Autodesk Inventor part; units mm, degrees
ref_plane "body_to_body2_XY" through (0, -15.2908, 0) normal (0, -1, 0) x (1, 0, 0)
ref_plane "body_to_body2_YZ" through (0, -15.2908, 0) normal (1, 0, 0) x (0, 0, 1)
ref_plane "body_to_body2_ZX" through (0, -15.2908, 0) normal (0, 0, 1) x (0, -1, 0)
sketch "Sketch_1" plane through (0, 0, 0) normal (0, 1, 0) x (-1, 0, 0)
  line L0 (9.7028, 14.4018) -> (-9.7028, 14.4018)
  line L1 (-9.7028, 14.4018) -> (-9.7028, -14.4018)
  line L2 (-9.7028, -14.4018) -> (9.7028, -14.4018)
  line L3 (9.7028, -14.4018) -> (9.7028, 14.4018)
extrude "Extrusion1" add sketch "Sketch_1" against normal blind 22.3012
sketch "Sketch_2" plane through (0, 0, 0) normal (0, 1, 0) x (-1, 0, 0)
  circle A0 centre (0, 0) radius 8.5725
extrude "Extrusion2" add sketch "Sketch_2" along normal blind 0.9906
sketch "Sketch_3" plane through (0, 0, 0) normal (1, 0, 0) x (0, 1, 0)
  line L0 (0.9906, 0) -> (9.6012, 0)
  line L1 (9.6012, 0) -> (9.6012, -4.9265)
  line L2 (9.6012, -4.9265) -> (8.5277, -6)
  line L3 (8.5277, -6) -> (0.9906, -6)
  line L4 (0.9906, -6) -> (0.9906, 0)
  line L5 (0.9906, 0) -> (9.6012, 0)
revolve "Revolution1" add sketch "Sketch_3" angle 360 about axis through (0, 0.9906, 0) along (0, 1, 0)
sketch "Sketch_10" plane through (0, 0.9906, 0) normal (0, 1, 0) x (1, 0, 0)
  line L0 (-2.9909, 5.2014) -> (2.9909, 5.2014)
  arc A0 (2.9909, 5.2014) -> (-2.9909, 5.2014) centre (0, 0) ccw
extrude "Extrusion3" cut sketch "Sketch_10" along normal blind 8.6106
sketch "Sketch5" plane through (0, 9.6012, 0) normal (0, 1, 0) x (1, 0, 0)
  point P0 (0, 0)
hole "Drilling 1" at (0, 9.6012, 0) direction (0, -1, 0) diameter 6 depth 8.6106 countersink diameter 8 countersink angle 90
sketch "Sketch_5" plane through (0, -22.3012, 0) normal (0, 1, 0) x (1, 0, 0)
  line L0 (-8.4328, -13.1318) -> (8.4328, -13.1318)
  line L1 (8.4328, -13.1318) -> (8.4328, 13.1318)
  line L2 (8.4328, 13.1318) -> (-8.4328, 13.1318)
  line L3 (-8.4328, 13.1318) -> (-8.4328, -13.1318)
extrude "Extrusion4" cut sketch "Sketch_5" along normal blind 0.254
sketch "Sketch_6" plane through (0, 0, -14.4018) normal (0, 0, 1) x (1, 0, 0)
  line L0 (-8.4328, -1.27) -> (-8.4328, -14.0208)
  line L1 (-8.4328, -14.0208) -> (8.4328, -14.0208)
  line L2 (8.4328, -14.0208) -> (8.4328, -1.27)
  line L3 (8.4328, -1.27) -> (-8.4328, -1.27)
extrude "Extrusion5" cut sketch "Sketch_6" along normal blind 0.254
sketch "Sketch_7" plane through (0, 0, 14.4018) normal (0, 0, 1) x (1, 0, 0)
  line L0 (-8.4328, -1.27) -> (-8.4328, -14.0208)
  line L1 (-8.4328, -14.0208) -> (8.4328, -14.0208)
  line L2 (8.4328, -14.0208) -> (8.4328, -1.27)
  line L3 (8.4328, -1.27) -> (-8.4328, -1.27)
extrude "Extrusion6" cut sketch "Sketch_7" against normal blind 0.254
sketch "Sketch_8" plane through (0, 0, 0) normal (1, 0, 0) x (0, 1, 0)
  line L0 (-17.3939, 15.113) -> (-18.4034, 15.113)
  line L1 (-18.4034, 15.113) -> (-18.796, 14.4018)
  line L2 (-18.796, 14.4018) -> (-17.3939, 14.4018)
  line L3 (-17.3939, 14.4018) -> (-17.3939, 15.113)
extrude "Extrusion7" add sketch "Sketch_8" along normal mid plane 2.54
sketch "Sketch_9" plane through (0, 0, 0) normal (1, 0, 0) x (0, 1, 0)
  line L0 (-17.3939, -14.4018) -> (-18.796, -14.4018)
  line L1 (-18.796, -14.4018) -> (-18.4034, -15.113)
  line L2 (-18.4034, -15.113) -> (-17.3939, -15.113)
  line L3 (-17.3939, -15.113) -> (-17.3939, -14.4018)
extrude "Extrusion8" add sketch "Sketch_9" along normal mid plane 2.54
ref_plane "body_to_body2_XY" through (0, -15.2908, 0) normal (0, -1, 0) x (1, 0, 0)
ref_plane "body_to_body2_YZ" through (0, -15.2908, 0) normal (1, 0, 0) x (0, 0, 1)
ref_plane "body_to_body2_ZX" through (0, -15.2908, 0) normal (0, 0, 1) x (0, -1, 0)
ref_plane "body_to_dummy_XY" through (0, 0, 0) normal (0, -1, 0) x (1, 0, 0)
ref_plane "body_to_dummy_YZ" through (0, 0, 0) normal (1, 0, 0) x (0, 0, 1)
ref_plane "body_to_dummy_ZX" through (0, 0, 0) normal (0, 0, 1) x (0, -1, 0)
ref_plane "body_to_terminal_XY" through (0, -22.3012, 0) normal (0, 1, 0) x (1, 0, 0)
ref_plane "body_to_terminal_YZ" through (0, -22.3012, 0) normal (1, 0, 0) x (0, 0, -1)
ref_plane "body_to_terminal_ZX" through (0, -22.3012, 0) normal (0, 0, -1) x (0, 1, 0)
ref_plane "body_to_toggle_XY" through (0, 2.4003, 0) normal (0, -1, 0) x (1, 0, 0)
ref_plane "body_to_toggle_YZ" through (0, 2.4003, 0) normal (1, 0, 0) x (0, 0, 1)
ref_plane "body_to_toggle_ZX" through (0, 2.4003, 0) normal (0, 0, 1) x (0, -1, 0)
ref_plane "body_to_washer_XY" through (0, 0.9906, 0) normal (0, -1, 0) x (1, 0, 0)
ref_plane "body_to_washer_YZ" through (0, 0.9906, 0) normal (1, 0, 0) x (0, 0, 1)
ref_plane "body_to_washer_ZX" through (0, 0.9906, 0) normal (0, 0, 1) x (0, -1, 0)
properties part number "WT_body"
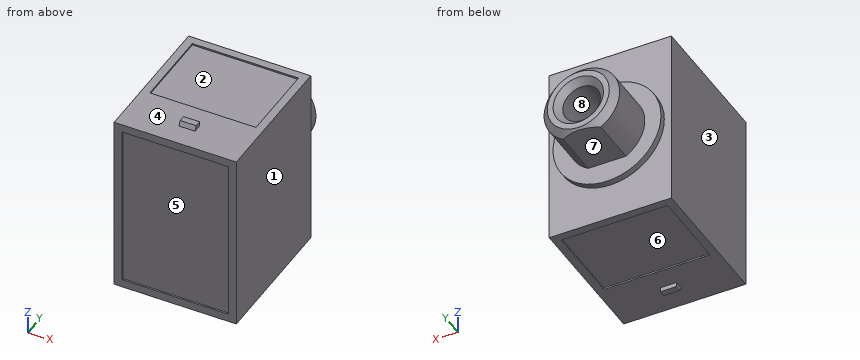
Input: part model. Units: mm. Frame: model coordinates. Face numbers are marked on the shaded views. A direction names the side the tool comes from. Give positions to 0.01 mm unless a question says otherwise; leave off trailing zeros. Order: outer loops, then holes, each group sorted by start corner. A loop starts at its lowest first (then second) coordinate and runs counter-clockwise, first axis right, second up. Notation, with made-up numbers: (76.5, 56) - (128.5, 56) arc R12 cw to (128.5, 69) - close; hole circle Ø5 at (80.5, 44.25). An arc over 180 degrees is marked (long way). Use a Markdown table: item, result.
(1) Line query: line 1 (X direction, y = 4, z = 0); line 2 (Z direction, x = 0, y = 2.5); line 3 (Z direction, x = -7.5, y = -14.5). Output: solid intervals per line, ascending. Write a range as from..to.
Computed values:
| item | result |
|---|---|
| line 1 | x = -6..-3, 3..6 |
| line 2 | z = -5.2..-3, 3..6 |
| line 3 | z = -14.4..14.4 |
(2) Section query C-C (x = 7). Output: boundary loops of the cut face in (y, z).
Computed values:
| item | result |
|---|---|
| outline | (-22.3, -14.4) - (-14.02, -14.4) - (-14.02, -14.15) - (-1.27, -14.15) - (-1.27, -14.4) - (0, -14.4) - (0, -4.95) - (0.99, -4.95) - (0.99, 4.95) - (0, 4.95) - (0, 14.4) - (-1.27, 14.4) - (-1.27, 14.15) - (-14.02, 14.15) - (-14.02, 14.4) - (-22.3, 14.4) - (-22.3, 13.13) - (-22.05, 13.13) - (-22.05, -13.13) - (-22.3, -13.13) - close |
(3) Section query D-D (y = -3). Output: boundary loops of the cut face in (x, z), then the cut area to 3 significant figures.
Computed values:
| item | result |
|---|---|
| outline | (-9.7, -14.4) - (-8.43, -14.4) - (-8.43, -14.15) - (8.43, -14.15) - (8.43, -14.4) - (9.7, -14.4) - (9.7, 14.4) - (8.43, 14.4) - (8.43, 14.15) - (-8.43, 14.15) - (-8.43, 14.4) - (-9.7, 14.4) - close |
| area | 550 mm2 |
(4) Pin query (flat end, axial travel): pin 1 (3 mm diameter, centred on y = 2, z = -7, fed in from -X); pin 2 (2 mm diameter, centred on x = 2.5, z = 11.5, fed in from -Y); pin 3 (1.8 mm diameter, centred on x = -1, y = 7, fed in from -Z). Return the tip coordinate at first contact, or that it passes through.
Computed values:
| item | result |
|---|---|
| pin 1 | stops at x = -6.23 |
| pin 2 | stops at y = -22.05 |
| pin 3 | stops at z = -5.2 |
(5) Section query B-B (y = 2). Output: boundary loops of the cut face in (x, z).
Computed values:
| item | result |
|---|---|
| outline | (-2.99, -5.2) - (2.99, -5.2) arc R6 ccw (long way) to start; hole circle Ø6 at (0, 0) |
(6) Access query for the marked faces 5, 6, 7 and 8. Directions: +Z, -Z, +X, -X, +Y, -Y. A direction counts if a zero-diameter tool reaches every point of the face in a straight line with its end or side. Return the directions, or none.
Computed values:
| item | result |
|---|---|
| face 5 | -Y |
| face 6 | -Z |
| face 7 | -Z, +X, -X, +Y |
| face 8 | +Y |
(7) Draft query along X for the marked faces 1, 2, 3 and 4. Return one class per face: released by +X, released by -X, zero draft, split by the parting line, or undercut.
Computed values:
| item | result |
|---|---|
| face 1 | released by +X |
| face 2 | undercut |
| face 3 | released by -X |
| face 4 | zero draft |
(8) Section query A-A (z = 0). Output: boundary loops of the cut face in (x, y).
Computed values:
| item | result |
|---|---|
| outline | (-9.7, -22.3) - (-8.43, -22.3) - (-8.43, -22.05) - (8.43, -22.05) - (8.43, -22.3) - (9.7, -22.3) - (9.7, 0) - (8.57, 0) - (8.57, 0.99) - (6, 0.99) - (6, 8.53) - (4.93, 9.6) - (4, 9.6) - (3, 8.6) - (3, 0.99) - (-3, 0.99) - (-3, 8.6) - (-4, 9.6) - (-4.93, 9.6) - (-6, 8.53) - (-6, 0.99) - (-8.57, 0.99) - (-8.57, 0) - (-9.7, 0) - close |
